The listing builds one solid part. Answer for the finished solid, in the listing's coordinates (mm). Face numbers are marked on the shaded views. A direction names the side the tool comes from. Give positions to 0.01 mm unless a question says otherwise; leave off trailing zeros. Loops run counter-clockwise (first coordinate to the right, second up) from the corner with the lowest first, then second, coordinate; pieces in that order, holes last. Notation, with made-up numbers: M 56.25,-39.5 L 106.25,-39.5 A17 ccw 106.25,-19.5 Z; hole C 30.25,-37.75 d2. An arc over 180 degrees is marked long. Use one line per item in the form item = value. Start each with the question number.
1. For the marked faces 1, 2 and 3, determine the directions among +Z, -Z, +X, -X, +Y, -Y from which every point of the face is accessible in a straight line to the end or side of a thin tool.
2. The part is cut by section B-B (y = -19). Write down the section's boundary in (x, z).
3. Straight lines are drawn through the part: line 1 (Y direction, x = 62, z = 2); line 2 (Z direction, x = 65.5, y = -10); line 3 (X direction, y = 21, z = 3.5). For each, find the intervals that lie inside material, in ascending order. Write a range as from..to.
4. The part is cut by section C-C (z = -3.5). Write down the section's boundary in (x, y), and give its area (3 significant figures).
5. Each of these flat-tipped pins is pushed along its axis until it touches: pin 1 Ø2.5 at (x, y) = (50.35, -7.98) entering from +Z; pin 2 Ø3 at (y, z) = (-30.5, 2) entering from -X; pin 3 Ø2 at (y, z) = (-43, -3.5) entering from +X; pin 4 Ø10.5 at (x, y) = (70, -19) entering from -Z. Where does it stop, or does it pass through?
6. The part is cut by section D-D (x = 75.5). Write down the section's boundary in (y, z).
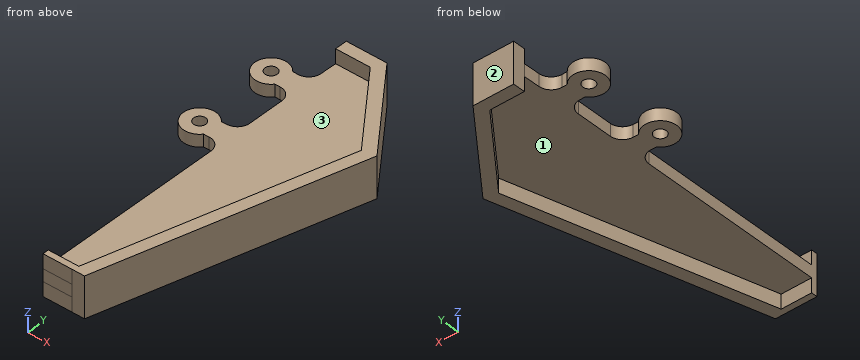
from build123d import *

# Parameters (mm, degrees)
BOSS_EXTRUDE4_DEPTH      = 5
BOSS_EXTRUDE4_DEPTH_BACK = 5
BOSS_EXTRUDE8_DEPTH      = 1.5
BOSS_EXTRUDE8_DEPTH_BACK = 1.5
BOSS_EXTRUDE9_START      = -6.5
BOSS_EXTRUDE9_DEPTH      = 10
SKETCH7_R                = 1.48
CUT_EXTRUDE4_DEPTH       = 3
SKETCH8_R                = 1.48
CUT_EXTRUDE5_DEPTH       = 3


with BuildPart() as part:
    # Sketch1 → Boss-Extrude4 (new, two sides: drawn at the far end of the back side and taken through both)
    with BuildSketch(Plane.XY.offset(-BOSS_EXTRUDE4_DEPTH_BACK)):
        Polygon((57.854367278, 21.520362054), (66.342730398, 21.520362054), (81.563363175, 1.615876121), (64.92491937, -60.479638348), (68.030747921, -60.479638348), (84.843243231, 2.265445145), (67.825274573, 24.520362054), (57.854367278, 24.520362054), align=None)
    extrude(amount=BOSS_EXTRUDE4_DEPTH + BOSS_EXTRUDE4_DEPTH_BACK)



with BuildPart() as body_2:
    # Sketch4 → Boss-Extrude8 (new, two sides: drawn at the far end of the back side and taken through both)
    with BuildSketch(Plane.XY.offset(-BOSS_EXTRUDE8_DEPTH_BACK)):
        with BuildLine():
            Line((57.854216238, 21.518374124), (66.342579359, 21.518374124))
            Line((66.342579359, 21.518374124), (81.563212135, 1.613888191))
            Line((81.563212135, 1.613888191), (64.92476833, -60.481626279))
            Line((64.92476833, -60.481626279), (57.854216238, -60.481626279))
            Line((57.854216238, -60.481626279), (57.854216238, -13.452758872))
            ThreePointArc((57.854216238, -13.452758872), (56.952658997, -11.308805051), (54.789857581, -10.453449291))
            Line((54.789857581, -10.453449291), (53.476715385, -10.481626465))
            ThreePointArc((53.476715385, -10.481626465), (46.354216528, -7.981626288), (53.476715385, -5.481626111))
            Line((53.476715385, -5.481626111), (54.850195116, -5.438621709))
            ThreePointArc((54.850195116, -5.438621709), (56.910567696, -4.527954069), (57.756309483, -2.440091154))
            Line((57.756309483, -2.440091154), (57.756309483, 6.518373554))
            ThreePointArc((57.756309483, 6.518373554), (56.877629826, 8.639693897), (54.756309483, 9.518373554))
            Line((54.756309483, 9.518373554), (53.476715385, 9.518373554))
            ThreePointArc((53.476715385, 9.518373554), (46.354216528, 12.018373731), (53.476715385, 14.518373908))
            Line((53.476715385, 14.518373908), (54.797976093, 14.518373908))
            ThreePointArc((54.797976093, 14.518373908), (56.904410545, 15.382271406), (57.797682695, 17.476417975))
            Line((57.797682695, 17.476417975), (57.854216238, 21.518374124))
        make_face()
    extrude(amount=BOSS_EXTRUDE8_DEPTH + BOSS_EXTRUDE8_DEPTH_BACK)


with BuildPart() as part_1:
    add(part.part)

    add(body_2.part)  # Boss-Extrude9 merges body 2
    # Sketch6 → Boss-Extrude9 (add)
    with BuildSketch(Plane.XY.offset(1.5).offset(BOSS_EXTRUDE9_START)):
        Polygon((57.854216238, -60.481626279), (57.854216238, -58.981626279), (65.326692139, -58.981626279), (64.92491937, -60.479638348), align=None)
    extrude(amount=BOSS_EXTRUDE9_DEPTH)

    # Sketch7 → Cut-Extrude4 (cut)
    with BuildSketch(Plane.XY.offset(1.5)):
        with Locations((50.354216528, -7.981626288)):
            Circle(SKETCH7_R)
    extrude(amount=-CUT_EXTRUDE4_DEPTH, mode=Mode.SUBTRACT)

    # Sketch8 → Cut-Extrude5 (cut)
    with BuildSketch(Plane.XY.offset(1.5)):
        with Locations((50.354216528, 12.018373731)):
            Circle(SKETCH8_R)
    extrude(amount=-CUT_EXTRUDE5_DEPTH, mode=Mode.SUBTRACT)


solid = part_1.part
Derived:
q1.face_1 = -Z, -X
q1.face_2 = +Z, -Z, +X, -X, +Y
q1.face_3 = +Z, -X
q2.outline = M 57.85,-1.5 L 76.04,-1.5 L 76.04,-5 L 79.15,-5 L 79.15,5 L 76.04,5 L 76.04,1.5 L 57.85,1.5 Z
q3.line_1 = -60.48..-58.98, 21.52..24.52
q3.line_2 = -1.5..1.5
q3.line_3 = 66.74..70.52
q4.outline = M 57.85,-60.48 L 64.92,-60.48 L 68.03,-60.48 L 84.84,2.27 L 67.83,24.52 L 57.85,24.52 L 57.85,21.52 L 66.34,21.52 L 81.56,1.62 L 65.33,-58.98 L 57.85,-58.98 Z
q4.area = 312 mm2
q5.pin_1 = through
q5.pin_2 = 57.85
q5.pin_3 = 72.98
q5.pin_4 = -1.5
q6.outline = M -32.6,-5 L -21.01,-5 L -21.01,-1.5 L 9.54,-1.5 L 9.54,1.5 L -21.01,1.5 L -21.01,5 L -32.6,5 Z; M 9.55,-5 L 14.48,-5 L 14.48,5 L 9.55,5 Z
